from build123d import *

# Parameters (mm, degrees)
F1_DEPTH = 50.8


with BuildPart() as f1:
    # F0 (on Front) → F1 (new body)
    with BuildSketch(Plane.XZ):
        with BuildLine():
            Line((58.541361, 3.749926), (26.791361, 3.749926))
            Line((26.791361, 3.749926), (26.791361, -21.650074))
            ThreePointArc((26.791361, -21.650074), (31.281489, -23.509946), (33.141361, -28.000074))
            Line((33.141361, -28.000074), (58.541361, -28.000074))
            Line((58.541361, -28.000074), (58.541361, 3.749926))
        make_face()
        with BuildLine():
            Line((26.791361, 3.749926), (7.741361, 3.749926))
            Line((7.741361, 3.749926), (7.741361, -28.000074))
            Line((7.741361, -28.000074), (20.441361, -28.000074))
            ThreePointArc((20.441361, -28.000074), (22.301233, -23.509946), (26.791361, -21.650074))
            Line((26.791361, -21.650074), (26.791361, 3.749926))
        make_face()
        with BuildLine():
            Line((20.441361, -28.000074), (7.741361, -28.000074))
            Line((7.741361, -28.000074), (7.741361, -47.050074))
            Line((7.741361, -47.050074), (26.791361, -47.050074))
            Line((26.791361, -47.050074), (26.791361, -34.350074))
            ThreePointArc((26.791361, -34.350074), (22.301233, -32.490202), (20.441361, -28.000074))
        make_face()
        with BuildLine():
            Line((58.541361, -47.050074), (58.541361, -28.000074))
            Line((58.541361, -28.000074), (33.141361, -28.000074))
            ThreePointArc((33.141361, -28.000074), (31.281489, -32.490202), (26.791361, -34.350074))
            Line((26.791361, -34.350074), (26.791361, -47.050074))
            Line((26.791361, -47.050074), (58.541361, -47.050074))
        make_face()
        Polygon((30.503648, 49.164883), (7.741361, 3.749926), (26.791361, 3.749926), (58.541361, 3.749926), align=None)
    extrude(amount=F1_DEPTH)


solid = f1.part
Input: part model. Units: mm. Frame: model coordinates. Give positions to 0.01 mm unless a question says otherwise; leave off trailing zeros. Write each loop counter-clockwise with the first axis right and the second up, starting at its lowest first coordinate (ties: lowest second). Pieces come first, ordered by that corner, then holes. Notation, with made-up numbers: (-23, 9.25) -> (9, 9.25) arc R27 ccw to (9, 28.25) -> close; hole circle Ø1 at (83.5, 38.25). An arc over 180 degrees is marked (long way). Use one line per item in the form item = value. Start each with the question number.
1) Draft query along Z for faces 1 (the flat face through (33, -50.8, -9)), 2 (the flat face through (33, -25, -47.05)), 3 (the flat face through (19.282, -25.044, 26.775)). Return one class per face: pulls with the +Z half, pulls with the -Z half, needs draft (parallel to the pull), parting line crosses it, or undercut.
2) Pin query (flat end, axial travel): pin 1 (5 mm diameter, centred on y = -29, z = 9, fed in from -X); pin 2 (2 mm diameter, centred on y = -9, z = 15, fed in from +X); pin 3 (5 mm diameter, centred on x = 37, y = -28, fed in from +Z). Return the tip coordinate at first contact, or that it passes through.
3) Section query C-C on x = 17.5. Return the cut outline in (y, z), then the cut area to 3 significant figures.
4) Ray query, probe 1 along Z at (x, y) = (24.5, -30); probe 2 along X at (y, z) = (-13.5, -24); probe 3 along Z at (x, y) = (13.5, -36). Return the intervals inside material, ascending. Write a range as from..to.
5) Section query A-A on y = -21. Return the cut outline in (x, z), then the cut area to 3 significant figures.
6) Section query B-B on z = 18. Return the cut outline in (x, y).
Outcome:
q1.face_1 = needs draft
q1.face_2 = pulls with the -Z half
q1.face_3 = pulls with the +Z half
q2.pin_1 = 9.12
q2.pin_2 = 52.21
q2.pin_3 = 42.69
q3.outline = (-50.8, -47.05) -> (0, -47.05) -> (0, 23.22) -> (-50.8, 23.22) -> close
q3.area = 3,570 mm^2
q4.probe_1 = -47.05..-33.92, -22.08..37.19
q4.probe_2 = 7.74..21.86, 31.72..58.54
q4.probe_3 = -47.05..15.24
q5.outline = (7.74, -47.05) -> (58.54, -47.05) -> (58.54, 3.75) -> (30.5, 49.16) -> (7.74, 3.75) -> close; hole circle Ø12.7 at (26.79, -28)
q5.area = 3,610 mm^2
q6.outline = (14.88, -50.8) -> (49.74, -50.8) -> (49.74, 0) -> (14.88, 0) -> close
